```python
from build123d import *

# Parameters (mm, degrees)
ZAOBLIT1_R    = 5
ZKOSEN_1_SIZE = 3


with BuildPart() as part:
    # Skica1 → Rotovat1 (revolve)
    with BuildSketch(Plane.XY, mode=Mode.PRIVATE) as rotovat1_sk:
        Polygon((0, 15), (0, 0), (70, 0), (70, 10), (55, 10), (55, 12), (50, 12), (50, 10), (46, 10), (46, 12), (40, 12), (40, 15), align=None)
    revolve(rotovat1_sk.sketch.rotate(Axis((-5.449862177, 0, 0), (1, 0, 0)), 90), axis=Axis((-5.449862177, 0, 0), (1, 0, 0)))

    # Zaoblit1
    zaoblit1_edges = [part.edges().sort_by_distance(p)[0] for p in [
        (70, 0, -10),
    ]]
    fillet(zaoblit1_edges, radius=ZAOBLIT1_R)

    # Zkosení1
    zkosen_1_edges = [part.edges().sort_by_distance(p)[0] for p in [
        (40, 0, -15),
    ]]
    chamfer(zkosen_1_edges, length=ZKOSEN_1_SIZE - 0.0001)  # a hair under: the kernel refuses the full size


solid = part.part
```
Input: part model. Units: mm. Frame: model coordinates. A direction names the side the tool comes from. Give positions to 0.01 mm unless a question says otherwise; leave off trailing zeros. Order: outer loops, then holes, each group sorted by start corner. A loop starts at its lowest first (then second) coordinate and runs counter-clockwise, first axis right, second up. Notation, with made-up numbers: (-8.75, 80.5) - (43.25, 80.5) arc R32 cw to (43.25, 119.5) - close; hole circle Ø7 at (9, 53.25). An arc over 180 degrees is marked (long way). Use a Markdown table: item, result.
(1) Pin query (flat end, axial travel): pin 1 (8 mm diameter, centred on x = 19, z = 6.5, fed in from -Y); pin 2 (5 mm diameter, centred on x = 62, y = 9.5, fed in from +Z); pin 3 (7 mm diameter, centred on y = -3, z = 4.5, fed in from +X); pin 4 (8 mm diameter, centred on x = 42, y = 6, fed in from +Z). Return the tip coordinate at first contact, or that it passes through.
Computed values:
| item | result |
|---|---|
| pin 1 | stops at y = -14.79 |
| pin 2 | stops at z = 7.14 |
| pin 3 | stops at x = 70 |
| pin 4 | stops at z = 12.96 |
(2) Section query A-A (x = 33). Output: boundary loops of the cut face in (y, z).
Computed values:
| item | result |
|---|---|
| outline | circle Ø30 at (0, 0) |
(3) Access query for faces 4 (the cylindrical face through (48, 0, -10)), 5 (the cylindrical face through (18.24, -12.65, 8.06)), 6 (the flat face through (55, -9, 5)). Directions: +Z, -Z, +X, -X, +Y, -Y. A direction counts if a zero-diameter tool reaches every point of the face in a straight line with its end or side. Return the directions, or none.
Computed values:
| item | result |
|---|---|
| face 4 | none |
| face 5 | +X, -X |
| face 6 | +X |
(4) Draft query along X for faces 1 (the flat face through (0, 0, 0)), 2 (the flat face through (50, -9, -5)), 3 (the flat face through (70, 0, 0)). Return one class per face: released by +X, released by -X, zero draft, split by the parting line, or undercut.
Computed values:
| item | result |
|---|---|
| face 1 | released by -X |
| face 2 | undercut |
| face 3 | released by +X |
(5) Line query: line 1 (X direction, y = -8.25, z = -6.75); line 2 (Z direction, x = 15, y = -0.5); line 3 (Z direction, x = 17.5, y = -5.25). Output: solid intervals per line, ascending. Write a range as from..to.
Computed values:
| item | result |
|---|---|
| line 1 | x = 0..46, 50..55 |
| line 2 | z = -14.99..14.99 |
| line 3 | z = -14.05..14.05 |
